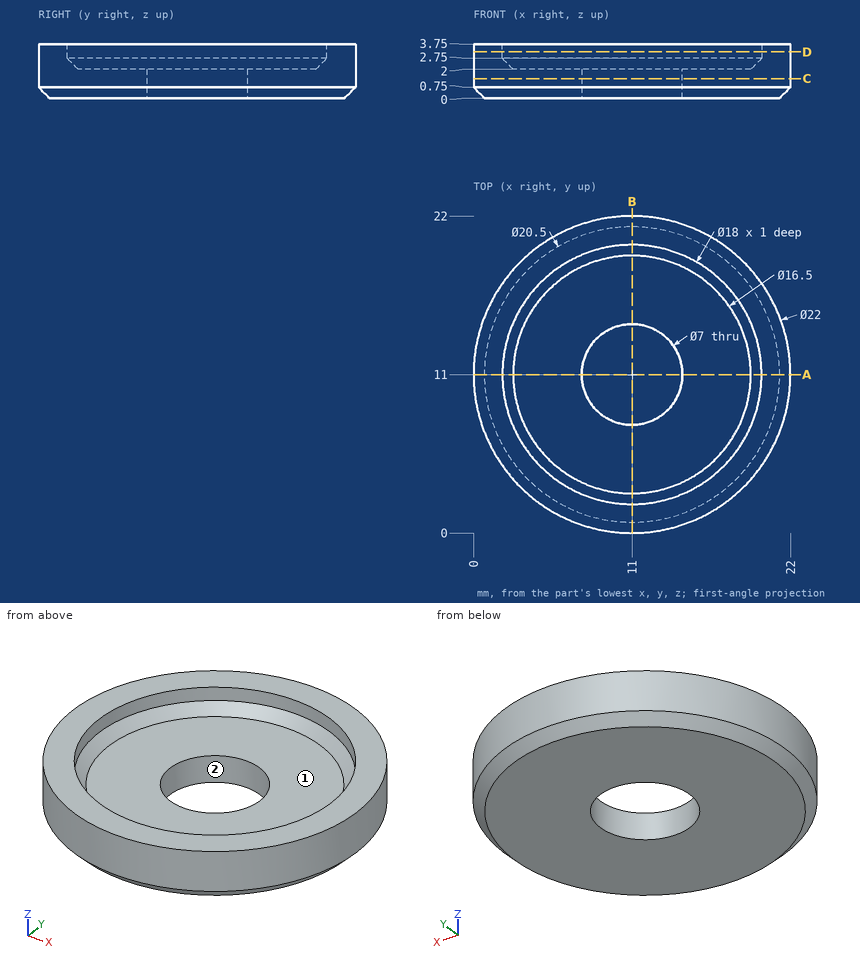
Verification items for this drawing (mm, ordinates from the low corner). A direction names the side the tool comes from. Give positions to 0.01 mm unless a question says otherwise; leave off trailing zeros. Write each loop counter-clockwise with the first axis right and the second up, starting at its lowest first coordinate (ties: lowest second). Pieces come first, ordered by that corner, then holes. Notation, with made-up numbers: (75.25, 18.25) -> (133.25, 18.25) arc R7 cw to (133.25, 25.25) -> close; hole circle Ø9 at (-39.5, 67). An arc over 180 degrees is marked (long way). Use one line per item in the form item = value.
Item 1: Sectioned sample at D-D on z = 3.2. Enter the section's corners in (x, y).
Results list:
outline = circle Ø22 at (11, 11); hole circle Ø18 at (11, 11)
Item 2: Depth check by flat-ended pin: pin 1 Ø2 at (x, z) = (15, 1.5) entering from +Y. Enter the tip coordinate at first touch or a pass-through.
Results list:
pin_1 = 21.58
Item 3: Sectioned sample at C-C on z = 1.35. Enter the section's corners in (x, y), plus the area to 3 significant figures.
Results list:
outline = circle Ø22 at (11, 11); hole circle Ø7 at (11, 11)
area = 342 mm2
Item 4: Scan lines: line 1 (Y direction, x = 11, z = 1.3); line 2 (Y direction, x = 11, z = 3.15); line 3 (Z direction, x = 7.5, y = 5.75). Record each from-to range of solid material in increasing order.
Results list:
line_1 = 0 to 7.5, 14.5 to 22
line_2 = 0 to 2, 20 to 22
line_3 = 0 to 2
Item 5: Access from +Z, -Z, +X, -X, +Y, -Y to the whole of each face (thin tool, end or side, straight path). Record for the marked faces 1 and 2.
Results list:
face_1 = +Z
face_2 = +Z, -Z
Item 6: Sectioned sample at A-A on y = 11. Enter the section's corners in (x, z).
Results list:
outline = (0, 0.75) -> (0.75, 0) -> (7.5, 0) -> (7.5, 2) -> (2.75, 2) -> (2, 2.75) -> (2, 3.75) -> (0, 3.75) -> close; (14.5, 0) -> (21.25, 0) -> (22, 0.75) -> (22, 3.75) -> (20, 3.75) -> (20, 2.75) -> (19.25, 2) -> (14.5, 2) -> close
